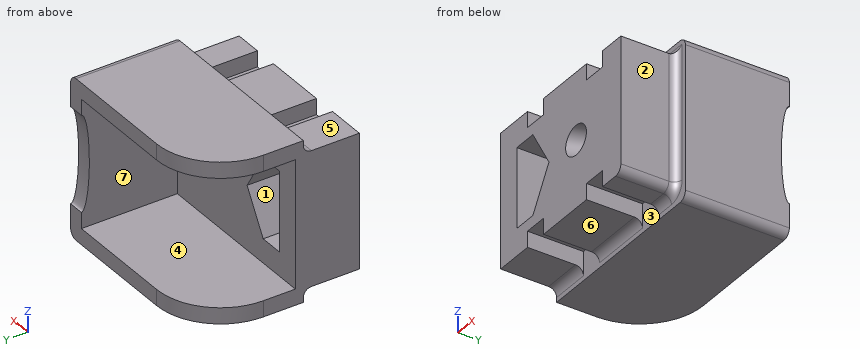
```python
from build123d import *

# Parameters (mm, degrees)
BOSS_EXTRUDE2_DEPTH = 2
SKETCH8_R           = 0.46
CUT_EXTRUDE1_DEPTH  = 6.857687257
CUT_EXTRUDE3_DEPTH  = 5.308421985
BOSS_EXTRUDE3_DEPTH = 0.5
SKETCH11_W          = 5
SKETCH11_H          = 5
BOSS_EXTRUDE4_DEPTH = 0.5
FILLET1_R           = 2
CUT_EXTRUDE5_DEPTH  = 1.75
SKETCH13_W          = 0.75
SKETCH13_H          = 1.75
CUT_EXTRUDE4_DEPTH  = 0.5
FILLET2_R           = 0.25
FILLET3_R           = 0.25
SKETCH15_RX         = 1.5
SKETCH15_RY         = 0.25
CUT_EXTRUDE6_DEPTH  = 8.158910532


with BuildPart() as part:
    # Sketch5 → Boss-Extrude2 (new body)
    with BuildSketch(Plane(origin=(0, 0, 0), x_dir=(1, 0, 0), z_dir=(0, 1, 0))):
        Polygon((-2.25, -2), (1.75, -2), (3.25, -2), (3.25, 2), (1.75, 2), (-2.25, 2), align=None)
    extrude(amount=-BOSS_EXTRUDE2_DEPTH)

    # Sketch8 → Cut-Extrude1 (cut, through all)
    with BuildSketch(Plane(origin=(0.85, 2.55, 0), x_dir=(0.948683298050514, -0.3162277660168378, 0), z_dir=(0.3162277660168378, 0.948683298050514, 0))):
        with Locations((1.829822128, 0)):
            Circle(SKETCH8_R)
    extrude(amount=-CUT_EXTRUDE1_DEPTH, mode=Mode.SUBTRACT)

    # Sketch12 → Cut-Extrude3 (cut, through all)
    with BuildSketch(Plane(origin=(0, 0, 0), x_dir=(1, 0, 0), z_dir=(0, 1, 0))):
        Polygon((-1.5, 1.25), (-1.5, -1.25), (-0.75, -1.25), (0, 0), (-0.75, 1.25), align=None)
    extrude(amount=-CUT_EXTRUDE3_DEPTH, mode=Mode.SUBTRACT)

    # Sketch10 → Boss-Extrude3 (add)
    with BuildSketch(Plane.XY.offset(2)):
        Polygon((3.25, -2), (3.25, 3), (-2.25, 3), (-2.25, 0), (-2.25, -2), align=None)
    boss_extrude3 = extrude(amount=BOSS_EXTRUDE3_DEPTH)

    # Mirror1: Boss-Extrude3 across plane
    add(boss_extrude3.mirror(Plane.XY))

    # Sketch11 → Boss-Extrude4 (add)
    with BuildSketch(Plane(origin=(3.25, 0, 0), x_dir=(0, 0, -1), z_dir=(1, 0, 0))):
        with Locations((0, 0.5)):
            Rectangle(SKETCH11_W, SKETCH11_H)
    extrude(amount=BOSS_EXTRUDE4_DEPTH)

    # Fillet1
    fillet1_edges = [part.edges().sort_by_distance(p)[0] for p in [
        (-2.25, 3, 2.25),
        (-2.25, 3, -2.25),
    ]]
    fillet(fillet1_edges, radius=FILLET1_R)

    # Sketch14 → Cut-Extrude5 (cut)
    with BuildSketch(Plane.XZ.offset(2)):
        Polygon((-2.25, 2.5), (-2.25, 2.1), (3.35, 2.1), (3.35, -2.1), (-2.25, -2.1), (-2.25, -2.5), (3.75, -2.5), (3.75, 2.5), align=None)
    extrude(amount=-CUT_EXTRUDE5_DEPTH, mode=Mode.SUBTRACT)

    # Sketch13 → Cut-Extrude4 (cut)
    with BuildSketch(Plane.XY.offset(2.1)):
        with Locations((-0.625, -1.125)):
            Rectangle(SKETCH13_W, SKETCH13_H)
        with Locations((2.125, -1.125)):
            Rectangle(SKETCH13_W, SKETCH13_H)
    cut_extrude4 = extrude(amount=-CUT_EXTRUDE4_DEPTH, mode=Mode.SUBTRACT)

    # Mirror2: Cut-Extrude4 across plane
    add(cut_extrude4.mirror(Plane.XY), mode=Mode.SUBTRACT)

    # Fillet2
    fillet2_edges = [part.edges().sort_by_distance(p)[0] for p in [
        (2.925, -0.25, -2.1),
        (3.35, -0.25, 0),
        (3.35, -1.125, -2.1),
        (-1.625, -0.25, 2.1),
        (0.75, -0.25, 2.1),
        (2.925, -0.25, 2.1),
        (0.75, -0.25, -2.1),
        (-1.625, -0.25, -2.1),
    ]]
    fillet(fillet2_edges, radius=FILLET2_R)

    # Fillet3
    fillet3_edges = [part.edges().sort_by_distance(p)[0] for p in [
        (3.75, 1.375, -2.5),
        (3.75, 1.375, 2.5),
    ]]
    fillet(fillet3_edges, radius=FILLET3_R)

    # Sketch15 → Cut-Extrude6 (cut, through all)
    with BuildSketch(Plane(origin=(3.75, 0, 0), x_dir=(0, 0, -1), z_dir=(1, 0, 0))):
        with Locations((0, 3)):
            Ellipse(SKETCH15_RX, SKETCH15_RY)
    extrude(amount=-CUT_EXTRUDE6_DEPTH, mode=Mode.SUBTRACT)


solid = part.part
```
Build history of the part. All positions in model axes, mm. Face numbers are marked on the shaded views. A direction names the side the tool comes from. Round coordinates to 2 decimals unless told otherwise and drop trailing zeros. Order: outer loops, then holes, each group sorted by start corner. A loop starts at its lowest first (then second) coordinate and runs counter-clockwise, first axis right, second up. Notation, with made-up numbers: (25, 52) -> (44, 52) arc R25 cw to (44, 64) -> close; hole circle Ø3 at (17.5, 2.25). An arc over 180 degrees is marked (long way). Answer in a Markdown table with one row per item.
1) Mould opens along Z. For the marked faces 5, 6 and 7 say: released by +Z, released by -Z, zero draft, split by the parting line, or undercut.
Values:
| item | result |
|---|---|
| face 5 | released by +Z |
| face 6 | released by -Z |
| face 7 | undercut |
2) Band-saw the part on C-C on y = 0.3. Give the cut face in (x, z).
Values:
| item | result |
|---|---|
| outline | (-2.25, -2.5) -> (3.5, -2.5) arc R0.25 ccw to (3.75, -2.25) -> (3.75, 2.25) arc R0.25 ccw to (3.5, 2.5) -> (-2.25, 2.5) -> (-2.25, 2) -> (3.25, 2) -> (3.25, -2) -> (-2.25, -2) -> close |
3) Band-saw the part on B-B on z = -1.75. Give the cut face in (x, y), and give its area (3 significant figures).
Values:
| item | result |
|---|---|
| outline | (-2.25, -2) -> (-1, -2) -> (-1, -0.25) -> (-0.25, -0.25) -> (-0.25, -2) -> (1.75, -2) -> (1.75, -0.25) -> (2.5, -0.25) -> (2.5, -2) -> (3.35, -2) -> (3.35, -0.5) arc R0.25 cw to (3.6, -0.25) -> (3.75, -0.25) -> (3.75, 3) -> (3.25, 3) -> (3.25, 0) -> (-2.25, 0) -> close |
| area | 10.2 mm2 |
4) Band-saw the part on D-D on x = 0.5. Give the cut face in (y, z).
Values:
| item | result |
|---|---|
| outline | (-2, -2.1) -> (-0.5, -2.1) arc R0.25 cw to (-0.25, -2.35) -> (-0.25, -2.5) -> (3, -2.5) -> (3, -2) -> (0, -2) -> (0, 2) -> (3, 2) -> (3, 2.5) -> (-0.25, 2.5) -> (-0.25, 2.35) arc R0.25 cw to (-0.5, 2.1) -> (-2, 2.1) -> close |
5) Band-saw the part on A-A on x = -1.25. Give the cut face in (y, z), and give its area (3 significant figures).
Values:
| item | result |
|---|---|
| outline | (-2, -2.1) -> (-0.5, -2.1) arc R0.25 cw to (-0.25, -2.35) -> (-0.25, -2.5) -> (2.73, -2.5) -> (2.73, -2) -> (0, -2) -> (0, -1.25) -> (-2, -1.25) -> close; (-2, 1.25) -> (0, 1.25) -> (0, 2) -> (2.73, 2) -> (2.73, 2.5) -> (-0.25, 2.5) -> (-0.25, 2.35) arc R0.25 cw to (-0.5, 2.1) -> (-2, 2.1) -> close |
| area | 6.36 mm2 |
6) Pin check, flat tips, straight feed: P1, Ø0.6, axis at x = -2, y = -1, coming from the +Z side; P2, Ø0.8, axis at x = 1, y = -1, coming from the -Z side; P3, Ø0.8, axis at y = -1.5, z = -2, coming from the +X side. Stop position of each tip, or through.
Values:
| item | result |
|---|---|
| P1 | z = 2.1 |
| P2 | z = -2.1 |
| P3 | x = 3.35 |
7) Wall check: L1, parallel to Z at x = 3, y = 1.5; L2, parallel to X at y = -1.05, z = 1.9; L3, parallel to X at y = -0.7, z = -0.2. Give the ranges that are in metal, low to high.
Values:
| item | result |
|---|---|
| L1 | -2.5 to -2, 2 to 2.5 |
| L2 | -2.25 to -1, -0.25 to 1.75, 2.5 to 3.35 |
| L3 | -2.25 to -1.5, -0.12 to 1.26, 2.13 to 3.35 |
8) Which spindle directions (+Z, -Z, +X, -X, +Y, -Y) get a long thin tool onto all of the face, cutting with end or side? Do the marked faces 1, 2, 3 and 4. Say none if no direction does.
Values:
| item | result |
|---|---|
| face 1 | +Y, -Y |
| face 2 | +Z, -Z, +X, -Y |
| face 3 | -Y |
| face 4 | -X, +Y |
